```python
from build123d import *

# Parameters (mm, degrees)
SKETCH_R           = 40
PAD_DEPTH          = 5
SKETCH001_R        = 7.5
SKETCH001_R_2      = 18
POCKET_DEPTH       = 5
POLARPATTERN_COUNT = 6
SKETCH002_R        = 16
SKETCH002_R_2      = 12.5
POCKET001_DEPTH    = 2
CHAMFER_SIZE       = 1
CHAMFER001_SIZE    = 1


with BuildPart() as part:
    # Sketch → Pad (new body)
    with BuildSketch(Plane.XY):
        Circle(SKETCH_R)
    extrude(amount=-PAD_DEPTH)

    # Sketch001 → Pocket (cut)
    with BuildSketch(Plane.XY):
        Circle(SKETCH001_R)
        with Locations((46.188, 0)):
            Circle(SKETCH001_R_2)
        with BuildLine():
            ThreePointArc((-2, 23.09), (0, 21.09), (2, 23.09))
            Line((2, 23.09), (2, 43.09))
            ThreePointArc((2, 43.09), (0, 45.09), (-2, 43.09))
            Line((-2, 43.09), (-2, 23.09))
        make_face()
    pocket = extrude(amount=-POCKET_DEPTH, mode=Mode.SUBTRACT)

    # PolarPattern: Pocket ×6 about axis
    polarpattern_axis = Axis((0, 0, 0), (0, 0, 1))
    for i in range(1, POLARPATTERN_COUNT):
        add(pocket.rotate(polarpattern_axis, i * 360 / POLARPATTERN_COUNT), mode=Mode.SUBTRACT)

    # Sketch002 → Pocket001 (cut)
    with BuildSketch(Plane.XY):
        Circle(SKETCH002_R)
        Circle(SKETCH002_R_2, mode=Mode.SUBTRACT)
    extrude(amount=-POCKET001_DEPTH, mode=Mode.SUBTRACT)

    # Chamfer
    chamfer_edges = [part.edges().sort_by_distance(p)[0] for p in [
        (-16, 0, 0),
        (-12.5, 0, 0),
    ]]
    chamfer(chamfer_edges, length=CHAMFER_SIZE)

    # Chamfer001
    chamfer001_edges = [part.edges().sort_by_distance(p)[0] for p in [
        (-28.188, 0, 0),
        (-28.297107, -14.027941, 0),
        (-18.264476, -10.545, 0),
        (-26.297107, -17.492043, 0),
        (-14.094, -24.411524, 0),
        (-2, -31.519984, 0),
        (0, -21.09, 0),
        (2, -31.519984, 0),
        (14.094, -24.411524, 0),
        (26.297107, -17.492043, 0),
        (18.264476, -10.545, 0),
        (28.297107, -14.027941, 0),
        (28.188, 0, 0),
        (28.297107, 14.027941, 0),
        (18.264476, 10.545, 0),
        (26.297107, 17.492043, 0),
        (14.094, 24.411524, 0),
        (2, 31.519984, 0),
        (0, 21.09, 0),
        (-2, 31.519984, 0),
        (-14.094, 24.411524, 0),
        (-26.297107, 17.492043, 0),
        (-18.264476, 10.545, 0),
        (-28.297107, 14.027941, 0),
    ]]
    chamfer(chamfer001_edges, length=CHAMFER001_SIZE)


solid = part.part
```
Geometry: final body of the model. Coordinates: model frame, mm. A direction names the side the tool comes from. Round coordinates to 2 decimals unless told otherwise and drop trailing zeros. Write each loop counter-clockwise with the first axis right and the second up, starting at its lowest first coordinate (ties: lowest second). Pieces come first, ordered by that corner, then holes.
Item 1: Section query A-A (x = 0). Return loops of the section in (y, z).
Item 2: Set-up query: faces 1 (the face through (14.32, -24.283, -2.972)), 2 (the face through (2, 31, -3)), 3 (the face through (-26.4, -17.55, -2.97)), 4 (the face through (28.441, 13.542, -0.507)). Return all of +Z, -Z, +X, -X, +Y, -Y with unobstructed straight access to the full face (end or side cutting, diameter ignored); none if empty.
Item 3: Material intervals for L1, parallel to Y at x = 0, z = -1.4; L2, parallel to Y at x = -19, z = -3.7; L3, parallel to Y at x = 25, z = -2.95, sorted ascending.
Item 4: Section query B-B (y = 0). Return loops of the section in (x, z), plus the area to 3 significant figures.
Item 5: Section query C-C (x = -30.5). Give the number of separate pieces and of enclosed holes in the cut face, plus the area to 3 significant figures.
Item 6: Mould query, pull axis X, two halves, no side actions, for faces 5 (the face through (28.19, 0.26, -2.97)), 6 (the face through (-36.27, 16.87, -2.46)), 7 (the face through (-28.195, -13.969, -2.972)). Classes: +X half, -X half, draft (parallel to the pull), parting line (faces both ways), or undercut.
Item 7: Pin query (flat end, axial travel): P1, Ø3, axis at x = 0, z = -3, coming from the -Y side; P2, Ø1.5, axis at x = 29.5, z = -3.5, coming from the -Y side; P3, Ø3, axis at y = 32, z = -2, coming from the -X side. Return the tip coordinate at first contact, or that it passes through.
Completed:
1. outline: (-21.09, -5) - (-7.5, -5) - (-7.5, 0) - (-11.5, 0) - (-12.5, -1) - (-12.5, -2) - (-16, -2) - (-16, -1) - (-17, 0) - (-20.09, 0) - (-21.09, -1) - close; (7.5, -5) - (21.09, -5) - (21.09, -1) - (20.09, 0) - (17, 0) - (16, -1) - (16, -2) - (12.5, -2) - (12.5, -1) - (11.5, 0) - (7.5, 0) - close
2. face 1: +Z, -Z, -Y
2. face 2: +Z, -Z, +Y
2. face 3: +Z, -Z
2. face 4: +Z
3. L1: y = -21.09 to -16, -12.5 to -7.5, 7.5 to 12.5, 16 to 21.09
3. L2: y = -22.47 to -13.28, -9.81 to 9.81, 13.28 to 22.47
3. L3: y = -22.1 to -16.74, -12.12 to 12.12, 16.74 to 22.1
4. outline: (-28.19, -5) - (-7.5, -5) - (-7.5, 0) - (-11.5, 0) - (-12.5, -1) - (-12.5, -2) - (-16, -2) - (-16, -1) - (-17, 0) - (-27.19, 0) - (-28.19, -1) - close; (7.5, -5) - (28.19, -5) - (28.19, -1) - (27.19, 0) - (17, 0) - (16, -1) - (16, -2) - (12.5, -2) - (12.5, -1) - (11.5, 0) - (7.5, 0) - close
4. area: 190 mm2
5. separate pieces: 4
5. enclosed holes: 0
5. area: 96.2 mm2
6. face 5: +X half
6. face 6: -X half
6. face 7: undercut
7. P1: stops at y = -21.77
7. P2: stops at y = -23.48
7. P3: stops at x = -7.81
